from build123d import *

# Parameters (mm, degrees)
SKETCH1_R           = 63.5
SKETCH1_R_2         = 34.925
SKETCH1_R_3         = 3.2639
BOSS_EXTRUDE1_DEPTH = 6.35


with BuildPart() as part:
    # Sketch1 → Boss-Extrude1 (new body)
    with BuildSketch(Plane(origin=(0, 0, 0), x_dir=(1, 0, 0), z_dir=(0, 1, 0))):
        Circle(SKETCH1_R)
        Circle(SKETCH1_R_2, mode=Mode.SUBTRACT)
        with Locations((0, 58.42)):
            Circle(SKETCH1_R_3, mode=Mode.SUBTRACT)
        with Locations((29.21, 50.593204089)):
            Circle(SKETCH1_R_3, mode=Mode.SUBTRACT)
        with Locations((50.593204089, 29.21)):
            Circle(SKETCH1_R_3, mode=Mode.SUBTRACT)
        with Locations((58.42, 0)):
            Circle(SKETCH1_R_3, mode=Mode.SUBTRACT)
        with Locations((50.593204089, -29.21)):
            Circle(SKETCH1_R_3, mode=Mode.SUBTRACT)
        with Locations((29.21, -50.593204089)):
            Circle(SKETCH1_R_3, mode=Mode.SUBTRACT)
        with Locations((0, -58.42)):
            Circle(SKETCH1_R_3, mode=Mode.SUBTRACT)
        with Locations((-29.21, -50.593204089)):
            Circle(SKETCH1_R_3, mode=Mode.SUBTRACT)
        with Locations((-50.593204089, -29.21)):
            Circle(SKETCH1_R_3, mode=Mode.SUBTRACT)
        with Locations((-58.42, 0)):
            Circle(SKETCH1_R_3, mode=Mode.SUBTRACT)
        with Locations((-50.593204089, 29.21)):
            Circle(SKETCH1_R_3, mode=Mode.SUBTRACT)
        with Locations((-29.21, 50.593204089)):
            Circle(SKETCH1_R_3, mode=Mode.SUBTRACT)
    extrude(amount=BOSS_EXTRUDE1_DEPTH)


solid = part.part
CAD build for the part. Positions are in the model's coordinates, mm. Round coordinates to 2 decimals unless told otherwise and drop trailing zeros. Write each loop counter-clockwise with the first axis right and the second up, starting at its lowest first coordinate (ties: lowest second). Pieces come first, ordered by that corner, then holes.
(1) Drop flat-ended pins along their axis: P1, Ø5, axis at x = -50.59, z = -29.21, coming from the +Y side; P2, Ø3, axis at x = -44, y = 5.5, coming from the -Z side; P3, Ø3, axis at x = -6, y = 5, coming from the +Z side; P4, Ø2, axis at y = 5.5, z = -29, coming from the -X side. Give the stop position or say it passes through.
(2) Slice it at C-C, the plane x = -16. Write the cut outline in (y, z), and give its area (3 significant figures).
(3) Mould opens along Z. For faces 1 (the face through (-13.77, 3.13, 61.99)), 2 (the face through (27, 6.35, 27)), 3 (the face through (-27.715, 3.131, 21.251)) say: pulls with the +Z half, pulls with the -Z half, needs draft (parallel to the pull), parting line crosses it, or undercut.
(4) Probe line 1 along X through (y, z) = (3.5, 0) (3 decimals); line 2 along Z through (x, y) = (-53, 5.5) (3 decimals); line 3 along X through (y, z) = (3, -29.21). List the from-to ranges inside material, lowest first.
(5) Slice it at D-D, the plane y = 5. Count the separate pieces of the cut face and the enclosed holes in it, and give its area (3 significant figures).
(6) Slice it at A-A, the plane x = 0. Write the cut outline in (y, z) (3 decimals), and give its area (3 significant figures).
(7) Slice it at B-B, the plane z = 29.21. Write the cut outline in (x, y), and give its area (3 significant figures).
From the geometry:
1. P1: passes through
1. P2: stops at z = -47.18
1. P3: stops at z = 63.34
1. P4: stops at x = -56.99
2. outline: (0, -61.45) - (6.35, -61.45) - (6.35, -31.04) - (0, -31.04) - close; (0, 31.04) - (6.35, 31.04) - (6.35, 61.45) - (0, 61.45) - close
2. area: 386 mm2
3. face 1: parting line crosses it
3. face 2: needs draft
3. face 3: undercut
4. line 1: x = -63.5 to -61.684, -55.156 to -34.925, 34.925 to 55.156, 61.684 to 63.5
4. line 2: z = -34.975 to -31.415, -27.005 to 27.005, 31.415 to 34.975
4. line 3: x = -56.38 to -53.86, -47.33 to -19.15, 19.15 to 47.33, 53.86 to 56.38
5. separate pieces: 1
5. enclosed holes: 13
5. area: 8,430 mm2
6. outline: (0, -63.5) - (6.35, -63.5) - (6.35, -61.684) - (0, -61.684) - close; (0, -55.156) - (6.35, -55.156) - (6.35, -34.925) - (0, -34.925) - close; (0, 34.925) - (6.35, 34.925) - (6.35, 55.156) - (0, 55.156) - close; (0, 61.684) - (6.35, 61.684) - (6.35, 63.5) - (0, 63.5) - close
6. area: 280 mm2
7. outline: (-56.38, 0) - (-53.86, 0) - (-53.86, 6.35) - (-56.38, 6.35) - close; (-47.33, 0) - (-19.15, 0) - (-19.15, 6.35) - (-47.33, 6.35) - close; (19.15, 0) - (47.33, 0) - (47.33, 6.35) - (19.15, 6.35) - close; (53.86, 0) - (56.38, 0) - (56.38, 6.35) - (53.86, 6.35) - close
7. area: 390 mm2
